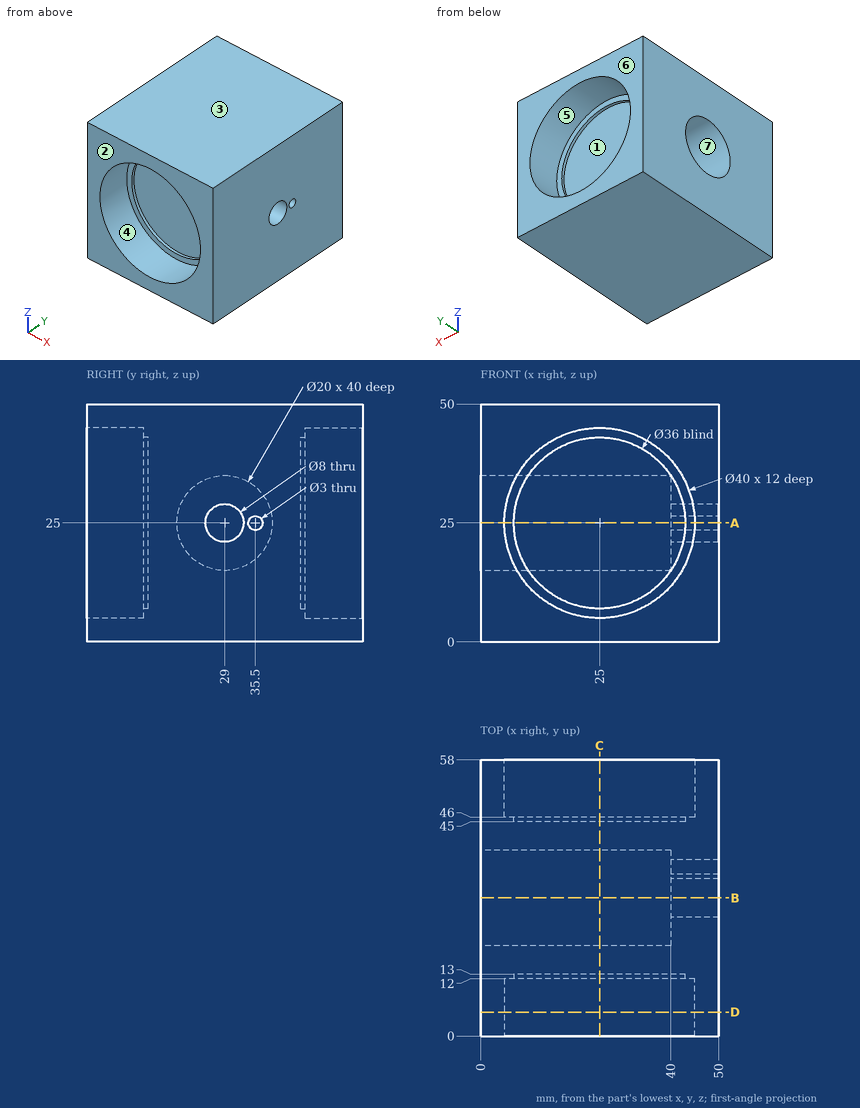
Print and shaded views of the part. All mm, measured from the part's lowest x, y and z. A direction names the side the tool comes from. Round coordinates to 2 decimals unless told otherwise and drop trailing zeros. Write each loop counter-clockwise with the first axis right and the second up, starting at its lowest first coordinate (ties: lowest second). Pieces come first, ordered by that corner, then holes. Notation, with made-up numbers: (59, 59.25) - (75, 59.25) arc R32 ccw to (75, 88.25) - close; hole circle Ø1 at (42.25, 45). An arc over 180 degrees is marked (long way). One line per item, written item: value.
(1) Cut at C-C, the plane x = 25. Give the cut face in (y, z).
Values follow:
outline: (0, 0) - (58, 0) - (58, 5) - (46, 5) - (46, 7) - (45, 7) - (45, 43) - (46, 43) - (46, 45) - (58, 45) - (58, 50) - (0, 50) - (0, 45) - (12, 45) - (12, 43) - (13, 43) - (13, 7) - (12, 7) - (12, 5) - (0, 5) - close; hole circle Ø20 at (29, 25)
(2) 3-axis set-ups, long thin cutter, end or side, ignore diameter. For the marked faces 4, 5, 6 and 7: which of +Z, -Z, +X, -X, +Y, -Y reach the whole face in a straight line?
Values follow:
face 4: -Y
face 5: +Y
face 6: +Z, -Z, +X, -X, +Y
face 7: -X
(3) Cut at D-D, the plane y = 5. Give the cut face in (x, z).
Values follow:
outline: (0, 0) - (50, 0) - (50, 50) - (0, 50) - close; hole circle Ø40 at (25, 25)
(4) Two-plate mould, pull along Z, no slides. Class the marked faces 1, 2 and 3: pulls with the +Z half, pulls with the -Z half, needs draft (parallel to the pull), parting line crosses it, or undercut.
Values follow:
face 1: undercut
face 2: needs draft
face 3: pulls with the +Z half
(5) Cut at B-B, the plane y = 29. Give the cut face in (x, z), plus the area to 3 significant figures.
Values follow:
outline: (0, 0) - (50, 0) - (50, 21) - (40, 21) - (40, 15) - (0, 15) - close; (0, 35) - (40, 35) - (40, 29) - (50, 29) - (50, 50) - (0, 50) - close
area: 1,620 mm²
(6) Wall check: probe 1 along X at (y, z) = (8, 25); probe 2 along Z at (x, y) = (25, 45.8). Give the ranges that are in metal, low to high.
Values follow:
probe 1: x = 0 to 5, 45 to 50
probe 2: z = 0 to 7, 43 to 50
(7) Drop flat-ended pins along their axis: P1, Ø1.5, axis at x = 31.5, z = 15, coming from the -Y side; P2, Ø11, axis at x = 26, z = 24.5, coming from the +Y side; P3, Ø20, axis at x = 34, z = 28.5, coming from the +Y side. Give the stop position or say it passes through.
Values follow:
P1: stops at y = 13
P2: stops at y = 45
P3: stops at y = 46
(8) Cut at A-A, the plane z = 25. Give the number of separate pieces and of enclosed holes in the cut face, plus the area to 3 significant figures.
Values follow:
separate pieces: 3
enclosed holes: 0
area: 958 mm²
